Solid Edge part; units mm, degrees
sketch "Sketch1" plane through (0, 0, 0) normal (0, -1, 0) x (1, 0, 0)
  circle A0 centre (0, 0) radius 25
extrude "Protrusion1" add sketch "Sketch1" against normal blind 10
sketch "Sketch2" plane through (0, 10, 0) normal (0, 1, 0) x (0, 0, 1)
  circle A0 centre (-22, 0) radius 1.6
extrude "Cutout1" cut sketch "Sketch2" against normal up to next
pattern_circular "Pattern1" count 6 over 360 about axis through (0, 10, 0) along (0, -1, 0) of "Cutout1"
sketch "Sketch3" plane through (0, 10, 0) normal (0, 1, 0) x (0, 0, 1)
  line L0 (-27.1295, -25) -> (30.6259, -25)
  line L1 (30.6259, -25) -> (30.6259, -23)
  line L2 (30.6259, -23) -> (-27.1295, -23)
  line L3 (-27.1295, -23) -> (-27.1295, -25)
  line L4 (-24.9621, 25) -> (24.2465, 25)
  line L5 (24.2465, 25) -> (24.2465, 23)
  line L6 (24.2465, 23) -> (-24.9621, 23)
  line L7 (-24.9621, 23) -> (-24.9621, 25)
  dimension "D1" = 30.6259
extrude "Cutout2" cut sketch "Sketch3" against normal up to next
sketch "Sketch4" plane through (0, 0, 0) normal (0, -1, 0) x (0, 0, -1)
  circle A0 centre (0, 0) radius 6.45
extrude "ExtrudedCutout_3" cut sketch "Sketch4" against normal blind 5
chamfer "Chamfer_1" distance 1.5 angle 45 1 edges at (0, 0, 6.45)
Could you check a few things on this model? Use its own coordinates, in mm. A direction names the side the tool comes from. Round coordinates to 2 decimals unless told otherwise and drop trailing zeros. Loops run counter-clockwise (first coordinate to the right, second up) from the corner with the lowest first, then second, coordinate; pieces in that order, holes last. Notation, with made-up numbers: (44.25, 8) - (77.25, 8) arc R23 ccw to (77.25, 42) - close; hole circle Ø9 at (-14.75, -13.5). An arc over 180 degrees is marked (long way). Write item = value, one per line.
1) Imagine slicing it at A-A (z = 0). Please give me the cut outline in (x, y).
Computed:
outline = (-23, 0) - (-7.95, 0) - (-6.45, 1.5) - (-6.45, 5) - (6.45, 5) - (6.45, 1.5) - (7.95, 0) - (23, 0) - (23, 10) - (-23, 10) - close
2) If we mould it in two halves opening along X, with no side actions, what happens to faces 1 (the flat face through (0, 10, 0)), 2 (the cylindrical face through (17.97, 5.07, -9.82)), 3 (the cylindrical face through (0.481, 5.07, -20.474)), 4 (the cylindrical face through (0, 5, -25))? For each: pulls with the +X half, pulls with the -X half, needs draft (parallel to the pull), parting line crosses it, or undercut.
Computed:
face_1 = needs draft
face_2 = undercut
face_3 = undercut
face_4 = parting line crosses it
3) Imagine slicing it at B-B (x = 0). Please give me the cut outline in (y, z).
Computed:
outline = (0, -25) - (10, -25) - (10, -23.6) - (0, -23.6) - close; (0, -20.4) - (10, -20.4) - (10, 20.4) - (0, 20.4) - (0, 7.95) - (1.5, 6.45) - (5, 6.45) - (5, -6.45) - (1.5, -6.45) - (0, -7.95) - close; (0, 23.6) - (10, 23.6) - (10, 25) - (0, 25) - close
4) I'm going to push flat-ended pins straight in: P1, Ø14, axis at x = 1.5, z = -2, coming from the -Y side; P2, Ø4, axis at x = -2.5, y = 8, coming from the +Z side (3 decimals). Where does each tip first touch, or does it pass through?
Computed:
P1 = 0
P2 = 24.995
5) On a 3-axis mill with a long thin cutter (end or side, diameter ignored), from which of +Z, -Z, +X, -X, +Y, -Y can I reach the whole of each face in a straight line? I mean faces 5 (the cylindrical face through (-0.481, 5.07, 20.474)), 6 (the cylindrical face through (-6.297, 3.226, 1.398)). Say none if no direction works.
Computed:
face_5 = +Y, -Y
face_6 = -Y
6) Imagine slicing it at C-C (y = 4.25). Please give me the cut outline in (x, z), and give its area (3 significant figures).
Computed:
outline = (-23, -9.8) arc R25 ccw to (23, -9.8) - (23, 9.8) arc R25 ccw to (-23, 9.8) - close; hole circle Ø3.2 at (-19.05, -11); hole circle Ø3.2 at (-19.05, 11); hole circle Ø12.9 at (0, 0); hole circle Ø3.2 at (0, -22); hole circle Ø3.2 at (0, 22); hole circle Ø3.2 at (19.05, -11); hole circle Ø3.2 at (19.05, 11)
area = 1,730 mm2
7) I need wall thicknesses on line 1 along Z through (x, y) = (-18.5, 3); line 2 along Z through (x, y) = (-18, 5.25); line 3 along X through (y, z) = (5, 11). Which ranges of each line are inside material? Lowest first, please. Write a range as from..to.
Computed:
line_1 = -16.82..-12.5, -9.5..9.5, 12.5..16.82
line_2 = -17.35..-12.21, -9.79..9.79, 12.21..17.35
line_3 = -22.45..-20.65, -17.45..17.45, 20.65..22.45
8) Imagine slicing it at D-D (z = -11). Please give me the cut outline in (x, y).
Computed:
outline = (-22.45, 0) - (-20.65, 0) - (-20.65, 10) - (-22.45, 10) - close; (-17.45, 0) - (17.45, 0) - (17.45, 10) - (-17.45, 10) - close; (20.65, 0) - (22.45, 0) - (22.45, 10) - (20.65, 10) - close
